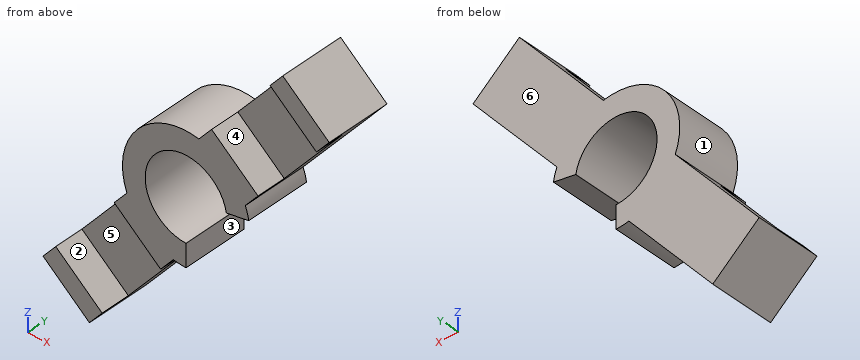
```python
from build123d import *

# Parameters (mm, degrees)
BOSS_EXTRUDE2_DEPTH = 8.55
SKETCH2_W           = 12
SKETCH2_H           = 3.872399236
CUT_EXTRUDE1_DEPTH  = 10


with BuildPart() as part:
    # Sketch1 → Boss-Extrude2 (new body)
    with BuildSketch(Plane(origin=(0, 0, 0), x_dir=(1, 0, 0), z_dir=(0, 1, 0))):
        with BuildLine():
            Line((0, 5.4), (0, 8.4))
            ThreePointArc((0, 8.4), (-0.846182507, 8.357270796), (-1.683756274, 8.229517896))
            Line((-1.683756274, 8.229517896), (-12.757091691, 21.426205161))
            Line((-12.757091691, 21.426205161), (-18.885447236, 16.283904283))
            Line((-18.885447236, 16.283904283), (-7.812111819, 3.087217019))
            ThreePointArc((-7.812111819, 3.087217019), (-6.434773322, -5.399415921), (1.683756274, -8.229517896))
            Line((1.683756274, -8.229517896), (12.757091691, -21.426205161))
            Line((12.757091691, -21.426205161), (18.885447236, -16.283904283))
            Line((18.885447236, -16.283904283), (7.812111819, -3.087217019))
            ThreePointArc((7.812111819, -3.087217019), (8.083367024, -2.284551937), (8.272385125, -1.458644692))
            Line((8.272385125, -1.458644692), (5.317961866, -0.937700159))
            ThreePointArc((5.317961866, -0.937700159), (-4.136639993, -3.471053092), (0, 5.4))
        make_face()
    extrude(amount=BOSS_EXTRUDE2_DEPTH)

    # Sketch2 → Cut-Extrude1 (cut)
    with BuildSketch(Plane(origin=(-3.064177772, 0, 2.571150439), x_dir=(0.64278761, 0, 0.766044443), z_dir=(-0.766044443, 0, 0.64278761))):
        with Locations((-16, 1.936199618)):
            Rectangle(SKETCH2_W, SKETCH2_H)
        with Locations((16, 1.936199618)):
            Rectangle(SKETCH2_W, SKETCH2_H)
    extrude(amount=-CUT_EXTRUDE1_DEPTH, mode=Mode.SUBTRACT)


solid = part.part
```
CAD build for the part. Positions are in the model's coordinates, mm. Face numbers are marked on the shaded views. A direction names the side the tool comes from. Round coordinates to 2 decimals unless told otherwise and drop trailing zeros. Write each loop counter-clockwise with the first axis right and the second up, starting at its lowest first coordinate (ties: lowest second). Pieces come first, ordered by that corner, then holes.
Item 1: Band-saw the part on C-C on z = 15.5. Write the cut outline in (x, y).
Filled in:
outline: (7.78, 3.87) - (15.75, 3.87) - (15.75, 0) - (18.23, 0) - (18.23, 8.55) - (7.78, 8.55) - close
Item 2: Drop flat-ended pins along their axis: pin 1 Ø4 at (y, z) = (3.5, -3) entering from -X; pin 2 Ø4 at (x, y) = (7, 4) entering from -Z; pin 3 Ø1 at (y, z) = (4.5, -16.5) entering from +X; pin 4 Ø9.5 at (x, z) = (0, 0) entering from -Y. Give the stop position or say it passes through.
Filled in:
pin 1: stops at x = -9.42
pin 2: stops at z = 0.94
pin 3: stops at x = -8.2
pin 4: passes through
Item 3: Band-saw the part on B-B on y = 6.75. Write the cut outline in (x, z), then the cut area to 3 significant figures.
Filled in:
outline: (-18.89, -16.28) - (-12.76, -21.43) - (-1.68, -8.23) arc R8.4 ccw to (0, -8.4) - (0, -5.4) arc R5.4 cw (long way) to (5.32, 0.94) - (8.27, 1.46) arc R8.4 ccw to (7.81, 3.09) - (18.89, 16.28) - (12.76, 21.43) - (1.68, 8.23) arc R8.4 ccw to (-7.81, -3.09) - close
area: 359 mm2
Item 4: Mould opens along Z. For the marked faces 1, 2 and 3 say: released by +Z, released by -Z, zero draft, split by the parting line, or undercut.
Filled in:
face 1: undercut
face 2: released by +Z
face 3: zero draft
Item 5: Tool access for the marked faces 4, 5 and 6: list every direction of +Z, -Z, +X, -X, +Y, -Y with a clear straight run to the whole face (end or side of a thin tool).
Filled in:
face 4: +Z, +X, -Y
face 5: -Y
face 6: +Z, -Z, +X, -X, +Y
Item 6: Drill centre lines: L1, parallel to X at y = 5, z = 0; L2, parallel to Y at x = -11, z = -8; L3, parallel to Z at x = -3, y = 4. Where is each one in solid material? Low to high.
Filled in:
L1: x = -8.4 to -5.4
L2: y = 3.87 to 8.55
L3: z = -9.8 to -4.49, 4.49 to 7.85
Item 7: Band-saw the part on D-D on x = -14.5. Write the cut outline in (y, z), then the cut area to 3 significant figures.
Filled in:
outline: (0, -19.96) - (8.55, -19.96) - (8.55, -11.06) - (3.87, -11.06) - (3.87, -16.55) - (0, -16.55) - close
area: 54.9 mm2
Item 8: Band-saw the part on A-A on y = 1.25. Write the cut outline in (x, z), then the cut area to 3 significant figures.
Filled in:
outline: (-18.89, -16.28) - (-12.76, -21.43) - (-11.08, -19.42) - (-17.21, -14.28) - close; (-9.49, -5.09) - (-3.36, -10.23) - (-1.68, -8.23) arc R8.4 ccw to (0, -8.4) - (0, -5.4) arc R5.4 cw (long way) to (5.32, 0.94) - (8.27, 1.46) arc R8.4 ccw to (7.81, 3.09) - (9.49, 5.09) - (3.36, 10.23) - (1.68, 8.23) arc R8.4 ccw to (-7.81, -3.09) - close; (11.08, 19.42) - (17.21, 14.28) - (18.89, 16.28) - (12.76, 21.43) - close
area: 167 mm2
